Design review of the part shown in the three views and the two pictorial views. Dimensions are in mm from the part's minimum x, y and z. Round coordinates to 2 decimals unless told otherwise and drop trailing zeros. Order: outer loops, then holes, each group sorted by start corner. A loop starts at its lowest first (then second) coordinate and runs counter-clockwise, first axis right, second up. Notation, with made-up numbers: (26.5, -39) - (40.5, -39) arc R21 ccw to (40.5, -20) - close; hole circle Ø8 at (43, 20). An arc over 180 degrees is marked (long way). Use CSV: the item, a comma, the result in double quotes.
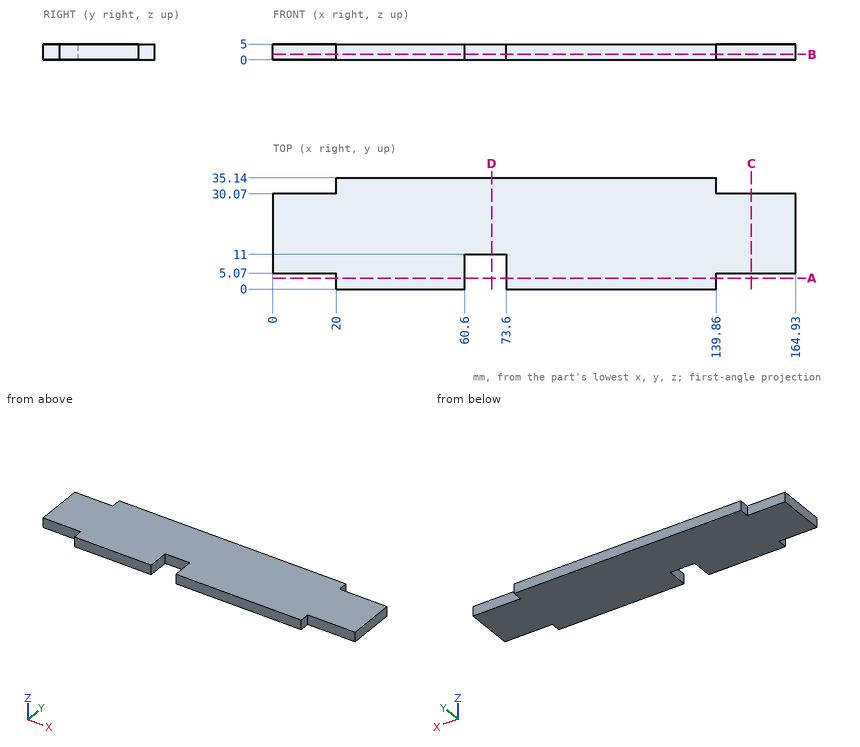
1) We need section C-C (x = 151). Give the boundary of the cut face in (y, z).
Data:
outline,"(5.07, 0) - (30.07, 0) - (30.07, 5) - (5.07, 5) - close"
2) Insertion check: pin 1 Ø1.5 at (x, z) = (148, 2) entering from +Y; pin 2 Ø2.5 at (y, z) = (3, 3) entering from +X; pin 3 Ø1.5 at (y, z) = (3, 2.5) entering from -X. Each pin has a flat end and moves straight along its axis. Give the tip position at first contact, or say it passes through.
Data:
pin 1,"stops at y = 30.07"
pin 2,"stops at x = 139.86"
pin 3,"stops at x = 20"
3) We need section A-A (y = 3.5). Give the boundary of the cut face in (x, z).
Data:
outline,"(20, 0) - (60.6, 0) - (60.6, 5) - (20, 5) - close; (73.6, 0) - (139.86, 0) - (139.86, 5) - (73.6, 5) - close"
4) To check wall thickness, follow L1, parallel to X at y = 10, z = 2.7; L2, parallel to X at y = 2, z = 1.15; L3, parallel to Y at x = 150.5, z = 4.6. State the ranges of each line that lie inside material, in increasing order. Write a range as from..to.
Data:
L1,"x = 0..60.6, 73.6..164.93"
L2,"x = 20..60.6, 73.6..139.86"
L3,"y = 5.07..30.07"
5) We need section D-D (x = 69). Give the boundary of the cut face in (y, z), then the cut area to 3 significant figures.
Data:
outline,"(11, 0) - (35.14, 0) - (35.14, 5) - (11, 5) - close"
area,"121 mm2"
6) We need section B-B (z = 1.7). Give the boundary of the cut face in (x, y).
Data:
outline,"(0, 5.07) - (20, 5.07) - (20, 0) - (60.6, 0) - (60.6, 11) - (73.6, 11) - (73.6, 0) - (139.86, 0) - (139.86, 5.07) - (164.93, 5.07) - (164.93, 30.07) - (139.86, 30.07) - (139.86, 35.14) - (20, 35.14) - (20, 30.07) - (0, 30.07) - close"
